from build123d import *

# Parameters (mm, degrees)
F2_SIZE2 = 2.54
F2_SIZE  = 2.54
F3_R     = 2.4384


with BuildPart() as f1:
    # F0 (on Front) → F1 (revolve)
    with BuildSketch(Plane.XZ):
        with BuildLine():
            Line((-50.8, 0), (0, 0))
            Line((0, 0), (0, 3.81))
            Line((0, 3.81), (-6.35, 3.81))
            Line((-6.35, 3.81), (-6.35, 2.0701))
            Line((-6.35, 2.0701), (-7.9502, 2.0701))
            Line((-7.9502, 2.0701), (-9.5504, 3.81))
            Line((-9.5504, 3.81), (-43.7388, 3.81))
            ThreePointArc((-43.7388, 3.81), (-46.037746, 4.762254), (-46.99, 7.0612))
            Line((-46.99, 7.0612), (-46.99, 19.05))
            Line((-46.99, 19.05), (-50.8, 19.05))
            Line((-50.8, 19.05), (-50.8, 0))
        make_face()
    revolve(axis=Axis((-25.4, 0, 0), (-1, 0, 0)))

    # F2
    f2_edges = [f1.edges().sort_by_distance(p)[0] for p in [
        (-46.99, 0, -19.05),
    ]]
    chamfer(f2_edges, length=F2_SIZE, length2=F2_SIZE2)

    # F3
    f3_edges = [f1.edges().sort_by_distance(p)[0] for p in [
        (0, 0, -3.81),
    ]]
    fillet(f3_edges, radius=F3_R)


solid = f1.part
Here's how the part is built. I have some questions about the finished solid (model axes, mm). A direction names the side the tool comes from. Coordinates: 2 decimals unless noted, no trailing zeros. Order: outer loops, then holes, each group sorted by start corner. A loop starts at its lowest first (then second) coordinate and runs counter-clockwise, first axis right, second up. Notation, with made-up numbers: M 60.25,30.25 L 95.25,30.25 A25 ccw 95.25,69.25 Z; hole C -38,23.5 d4. An arc over 180 degrees is marked long. Answer as CSV lines item,"result". Start each with the question number.
1. We'd pull the mould along X, two halves only. Please class faces 1 (the flat face through (-50.8, 0, 0)), 2 (the flat face through (-6.35, -2, 2)), 3 (the flat face through (-46.99, -3, -7)), 4 (the cylindrical face through (-50.17, -11.59, -15.12)): released by +X, released by -X, zero draft, split by the parting line, or undercut.
2. On a 3-axis mill with a long thin cutter (end or side, diameter ignored), from which of +Z, -Z, +X, -X, +Y, -Y can I reach the whole of each face in a straight line? I mean faces 5 (the flat face through (0, 0, 0)), 6 (the cylindrical face through (-26.88, -3.72, -0.83)), 7 (the cylindrical face through (-7.161, 1.399, -1.526)). Say none if no direction works.
3. I need wall thicknesses on line 1 (X direction, y = 8, z = 1); line 2 (X direction, y = 2.5, z = -1); line 3 (X direction, y = 4.5, z = 0). Which ranges of each line are inside material? Lowest first, please. Write a range as [from, to].
4. For pin 1 (10 mm diameter, centred on y = -6, z = 7, fed in from +X); pin 2 (8 mm diameter, centred on x = -8, y = -4.5, fed in from +Z); pin 3 (5 mm diameter, centred on y = 14, z = 11.5, fed in from +X), each with a flat end and sliding along its axis, tell me the tip position at first contact or that it passes through.
5. I want a section at A-A, the plane x = -16. Write out the boundary of the cut face in (y, z), and give its area (3 significant figures).
Recorded:
1,face 1,"released by -X"
1,face 2,"undercut"
1,face 3,"released by +X"
1,face 4,"zero draft"
2,face 5,"+Z, -Z, +X, +Y, -Y"
2,face 6,"+X"
2,face 7,"none"
3,line 1,"x = [-50.8, -46.99]"
3,line 2,"x = [-50.8, -8.52], [-6.35, -0.39]"
3,line 3,"x = [-50.8, -45.74]"
4,pin 1,"stops at x = -45.32"
4,pin 2,"stops at z = 3.72"
4,pin 3,"stops at x = -46.99"
5,outline,"C 0,0 d7.62"
5,area,"45.6 mm2"
